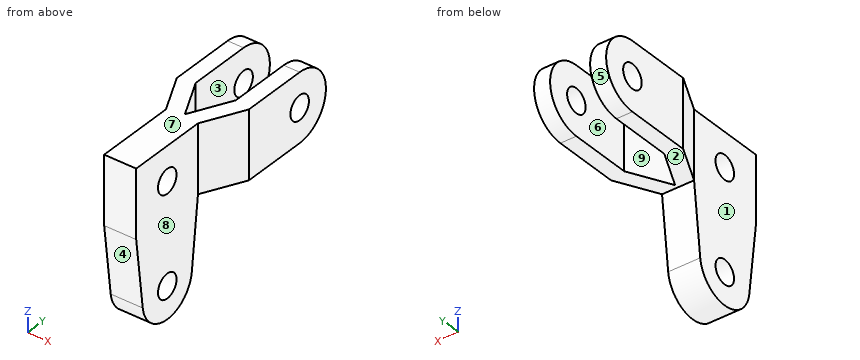
```python
from build123d import *

# Parameters (mm, degrees)
BASE_EXTRUDE_DEPTH  = 10.795
SKETCH2_R           = 1.905
CUT_EXTRUDE1_DEPTH  = 36.062279171
FILLET1_R           = 5.3975
SKETCH3_R           = 1.905
CUT_EXTRUDE2_DEPTH  = 35.159384445
BOSS_EXTRUDE1_START = -5.08
SKETCH4_R           = 1.905
BOSS_EXTRUDE1_DEPTH = 5.08


with BuildPart() as part:
    # Sketch1 → Base-Extrude (new body)
    with BuildSketch(Plane.XY):
        Polygon((-3.175, 3.549757914), (-5.715, 3.549757914), (-5.715, -12.289854749), (-2.54, -18.639854749), (-2.54, -31.339854749), (2.54, -31.339854749), (2.54, -18.639854749), (5.715, -12.289854749), (5.715, 3.549757914), (3.175, 3.549757914), (3.175, -11.690242086), (0, -18.040242086), (-3.175, -11.690242086), align=None)
    extrude(amount=BASE_EXTRUDE_DEPTH)

    # Sketch2 → Cut-Extrude1 (cut, through all)
    with BuildSketch(Plane(origin=(5.715, 0, 0), x_dir=(0, 0, -1), z_dir=(1, 0, 0))):
        with Locations(Location((-5.3975, -1.847742086, 0), (0, 0, 90))):
            Circle(SKETCH2_R)
    extrude(amount=-CUT_EXTRUDE1_DEPTH, mode=Mode.SUBTRACT)

    # Fillet1
    # the kernel refuses this fillet: 5.3975 mm, written as the material it takes off along each edge
    with BuildSketch(Plane(origin=(19.20875, 3.549757914, 0), x_dir=(0, -1, 0), z_dir=(-1, 0, 0)), Plane(origin=(10.31875, 3.549757914, 10.795), x_dir=(0, 0, -1), z_dir=(-1, 0, 0))) as fillet1_piece_1:
        with BuildLine():
            CenterArc((FILLET1_R, FILLET1_R), FILLET1_R, 180, 90)
            Line((0, FILLET1_R), (0, 0))
            Line((0, 0), (FILLET1_R, 0))
        make_face()
    extrude(amount=29.5275, mode=Mode.SUBTRACT)
    with BuildSketch(Plane(origin=(10.31875, 3.549757914, 0), x_dir=(0, 0, 1), z_dir=(-1, 0, 0)), Plane(origin=(19.20875, 3.549757914, 10.795), x_dir=(0, -1, 0), z_dir=(-1, 0, 0))) as fillet1_piece_2:
        with BuildLine():
            CenterArc((FILLET1_R, -FILLET1_R), FILLET1_R, 90, 90)
            Line((0, -FILLET1_R), (0, 0))
            Line((0, 0), (FILLET1_R, 0))
        make_face()
    extrude(amount=29.5275, mode=Mode.SUBTRACT)

    # Sketch3 → Cut-Extrude2 (cut, through all)
    with BuildSketch(Plane(origin=(2.54, 0, 0), x_dir=(0, 0, -1), z_dir=(1, 0, 0))):
        with Locations(Location((-5.3975, -24.951582086, 0), (0, 0, 90))):
            Circle(SKETCH3_R)
    extrude(amount=-CUT_EXTRUDE2_DEPTH, mode=Mode.SUBTRACT)

    # Sketch4 → Boss-Extrude1 (add)
    with BuildSketch(Plane(origin=(2.54, 0, 0), x_dir=(0, 0, -1), z_dir=(1, 0, 0)).offset(BOSS_EXTRUDE1_START)):
        with BuildLine():
            Line((0, -31.339854749), (11.146934896, -29.995009323))
            ThreePointArc((11.146934896, -29.995009323), (15.618430773, -24.934350077), (11.112705191, -19.904142887))
            Line((11.112705191, -19.904142887), (0, -18.639854749))
            Line((0, -18.639854749), (0, -31.339854749))
        make_face()
        with Locations(Location((10.53846, -24.951582086, 0), (0, 0, 90))):
            Circle(SKETCH4_R, mode=Mode.SUBTRACT)
    extrude(amount=BOSS_EXTRUDE1_DEPTH)


solid = part.part
```
Geometry: final body of the model. Coordinates: model frame, mm. Face numbers are marked on the shaded views. A direction names the side the tool comes from. Coordinates: 2 decimals unless noted, no trailing zeros. Order: outer loops, then holes, each group sorted by start corner. A loop starts at its lowest first (then second) coordinate and runs counter-clockwise, first axis right, second up. Notation, with made-up numbers: (39.25, 89) - (54.25, 89) arc R19 ccw to (54.25, 110) - close; hole circle Ø2 at (42, -14). An arc over 180 degrees is marked (long way). Write each question's results on one line, items separated by ' | '.
(1) Section query C-C, the plane z = -9.75. Return the cut outline in (x, y).
Values found:
outline: (-2.54, -30.16) - (2.54, -30.16) - (2.54, -26.69) - (-2.54, -26.69) - close; (-2.54, -23.22) - (2.54, -23.22) - (2.54, -19.75) - (-2.54, -19.75) - close
(2) Mould query, pull axis X, two halves, no side actions, for the marked faces 6, 7, 8 and 9. Classes: +X half, -X half, draft (parallel to the pull), parting line (faces both ways), or undercut.
Values found:
face 6: undercut | face 7: draft | face 8: +X half | face 9: undercut
(3) Line query: line 1 (Z direction, x = 2.25, y = -25) (3 decimals); line 2 (Y direction, x = -1.25, z = 4.5); line 3 (Y direction, x = 2.25, z = 6). Output: solid intervals per line, ascending. Write a range as [from, to].
Values found:
line 1: z = [-15.618, -12.443], [-8.634, 3.493], [7.302, 10.795] | line 2: y = [-31.34, -26.63], [-23.27, -15.54] | line 3: y = [-31.34, -26.76], [-23.14, -13.54]
(4) Section query A-A, the plane y = -11. Return the cut outline in (x, z) (3 decimals), plus the area to 3 significant figures.
Values found:
outline: (-5.715, 0) - (-3.175, 0) - (-3.175, 10.795) - (-5.715, 10.795) - close; (3.175, 0) - (5.715, 0) - (5.715, 10.795) - (3.175, 10.795) - close | area: 54.8 mm²
(5) Section query B-B, the plane z = 4.5. Return the cut outline in (x, y) (3 decimals), plus the area to 3 significant figures.
Values found:
outline: (-5.715, -12.29) - (-2.54, -18.64) - (-2.54, -23.271) - (2.54, -23.271) - (2.54, -18.64) - (5.715, -12.29) - (5.715, -3.528) - (3.175, -3.528) - (3.175, -11.69) - (0, -18.04) - (-3.175, -11.69) - (-3.175, -3.528) - (-5.715, -3.528) - close; (-5.715, -0.167) - (-3.175, -0.167) - (-3.175, 3.475) - (-5.715, 3.475) - close; (-2.54, -31.34) - (2.54, -31.34) - (2.54, -26.632) - (-2.54, -26.632) - close; (3.175, -0.167) - (5.715, -0.167) - (5.715, 3.475) - (3.175, 3.475) - close | area: 147 mm²
(6) First-contact query: pin 1 Ø2 at (x, y) = (0.5, -2.5) entering from -Z; pin 2 Ø5.5 at (x, y) = (2, -14) entering from -Z; pin 3 Ø14 at (y, z) = (-22.5, 0.5) entering from -X; pin 4 Ø4.5 at (y, z) = (-24.95, 5.4) entering from +X. Flat tips, straight axial feed; report the tip coordinate or a pass-through.
Values found:
pin 1: passes through | pin 2: stops at z = 0 | pin 3: stops at x = -4.11 | pin 4: stops at x = 2.54
(7) Set-up query: the marked faces 1, 2, 3, 4 and 5. Return all of +Z, -Z, +X, -X, +Y, -Y with unobstructed straight access to the full face (end or side cutting, diameter ignored); none if empty.
Values found:
face 1: +Z, -Z, -X, -Y | face 2: -Z, +X, -X, +Y | face 3: +Z, -Z, +Y | face 4: -Z, +X, -X, -Y | face 5: +X, -X, +Y
(8) Section query D-D, the plane x = -5. Return the cut outline in (y, z) (1 decimal), plus the area to 3 significant figures.
Values found:
outline: (-13.7, 0) - (-1.8, 0) arc R5.4 ccw to (-1.8, 10.8) - (-13.7, 10.8) - close; hole circle Ø3.8 at (-1.8, 5.4) | area: 163 mm²
